```python
from build123d import *

# Parameters (mm, degrees)
SKETCH_1_R      = 1.5
EXTRUDE_1_DEPTH = 1.5
EXTRUDE_2_DEPTH = 5
SKETCH_3_R      = 6
EXTRUDE_3_DEPTH = 3
SKETCH_4_R      = 4
EXTRUDE_4_DEPTH = 5


with BuildPart() as part:
    # 草图1 → 凸台-拉伸1 (new body)
    with BuildSketch(Plane(origin=(0, 0, 0), x_dir=(1, 0, 0), z_dir=(0, 1, 0))):
        with BuildLine():
            Line((-11, 13.5), (11, 13.5))
            ThreePointArc((11, 13.5), (14.535533906, 12.035533906), (16, 8.5))
            Line((16, 8.5), (16, -5.5))
            ThreePointArc((16, -5.5), (13.656854249, -11.156854249), (8, -13.5))
            Line((8, -13.5), (-8, -13.5))
            ThreePointArc((-8, -13.5), (-13.656854249, -11.156854249), (-16, -5.5))
            Line((-16, -5.5), (-16, 8.5))
            ThreePointArc((-16, 8.5), (-14.535533906, 12.035533906), (-11, 13.5))
        make_face()
        with Locations(Location((-13.4, 8.5, 0), (0, 0, 270))):
            Circle(SKETCH_1_R, mode=Mode.SUBTRACT)
        with Locations(Location((13.5, 8.5, 0), (0, 0, 270))):
            Circle(SKETCH_1_R, mode=Mode.SUBTRACT)
        with Locations(Location((-13.4, -2.93, 0), (0, 0, 270))):
            Circle(SKETCH_1_R, mode=Mode.SUBTRACT)
        with Locations(Location((13.5, -2.93, 0), (0, 0, 270))):
            Circle(SKETCH_1_R, mode=Mode.SUBTRACT)
    extrude(amount=EXTRUDE_1_DEPTH)

    # 草图2 → 凸台-拉伸2 (add)
    with BuildSketch(Plane(origin=(0, 1.5, 0), x_dir=(1, 0, 0), z_dir=(0, 1, 0))):
        Polygon((-9, 11.5), (9, 11.5), (11, 9.5), (11, -5.5), (9, -7.5), (-9, -7.5), (-11, -5.5), (-11, 9.5), align=None)
    extrude(amount=EXTRUDE_2_DEPTH)

    # 草图3 → 凸台-拉伸3 (add)
    with BuildSketch(Plane(origin=(0, 6.5, 0), x_dir=(1, 0, 0), z_dir=(0, 1, 0))):
        with Locations(Location((0, 3.5, 0), (0, 0, 270))):
            Circle(SKETCH_3_R)
    extrude(amount=EXTRUDE_3_DEPTH)

    # 草图4 → 凸台-拉伸4 (add)
    with BuildSketch(Plane(origin=(0, 9.5, 0), x_dir=(1, 0, 0), z_dir=(0, 1, 0))):
        with Locations(Location((0, 3.5, 0), (0, 0, 270))):
            Circle(SKETCH_4_R)
    extrude(amount=EXTRUDE_4_DEPTH)


solid = part.part
```
Geometry: final body of the model. Coordinates: model frame, mm. A direction names the side the tool comes from. Round coordinates to 2 decimals unless told otherwise and drop trailing zeros. Order: outer loops, then holes, each group sorted by start corner. A loop starts at its lowest first (then second) coordinate and runs counter-clockwise, first axis right, second up. Notation, with made-up numbers: (-19, -39.75) - (30, -39.75) arc R14 ccw to (30, -23.75) - close; hole circle Ø10 at (22, -39). An arc over 180 degrees is marked (long way). Write item = value, one per line. Start each with the question number.
Q1. Cut plane C-C on x = 0. Return the cut outline in (y, z).
Q2. Ray query, line 1 (X direction, y = 0.85, z = -8.5); line 2 (Z direction, x = -12.5, y = 1); line 3 (Y direction, x = -10, z = -6). Return the intervals inside material, ascending. Write a range as from..to.
Q3. Cut plane A-A on y = 1. Return the cut outline in (x, z), and give its area (3 significant figures).
Q4. Pin query (flat end, axial travel): pin 1 (1.5 mm diameter, centred on y = 7, z = 4, fed in from -X); pin 2 (4 mm diameter, centred on y = 4, z = -2.5, fed in from +X); pin 3 (5.5 mm diameter, centred on x = -1.5, y = 4.5, fed in from -Z). Return the tip coordinate at first contact, or that it passes through.
Q5. Cut plane D-D on z = -3.5. Return the cut outline in (x, y), and give its area (3 significant figures).
Q6. Cut plane B-B on z = 2.93. Return the cut outline in (x, y).
Q7. Pull-direction query (X, two-part tool) for faces 6 (the cylindrical face through (-14.57, 0.74, -12)), 7 (the cylindrical face through (13.719, 0.74, 11.094)), 8 (the flat face through (0, 4, -11.5)), 9 (the cylindrical face through (13.57, 0.74, -10)); classes: +X half, -X half, draft (parallel to the pull), parting line (faces both ways), or undercut.
Q8. Access query for faces 1 (the flat face through (-11, 4, -2)), 2 (the flat face through (-10, 4, 6.5)), 3 (the flat face through (-10, 4, -10.5)), 4 (the flat face through (11, 4, -2)), 5 (the cylindrical face through (-2.4, 12, -6.7)). Directions: +Z, -Z, +X, -X, +Y, -Y. A direction counts if a zero-diameter tool reaches every point of the face in a straight line with its end or side. Return the directions, or none.
Outcome:
q1.outline = (0, -13.5) - (1.5, -13.5) - (1.5, -11.5) - (6.5, -11.5) - (6.5, -9.5) - (9.5, -9.5) - (9.5, -7.5) - (14.5, -7.5) - (14.5, 0.5) - (9.5, 0.5) - (9.5, 2.5) - (6.5, 2.5) - (6.5, 7.5) - (1.5, 7.5) - (1.5, 13.5) - (0, 13.5) - close
q2.line_1 = -16..-14.9, -11.9..12, 15..16
q2.line_2 = -13.27..-9.7, -7.3..1.73, 4.13..12.11
q2.line_3 = 0..6.5
q3.outline = (-16, -8.5) arc R5 ccw to (-11, -13.5) - (11, -13.5) arc R5 ccw to (16, -8.5) - (16, 5.5) arc R8 ccw to (8, 13.5) - (-8, 13.5) arc R8 ccw to (-16, 5.5) - close; hole circle Ø3 at (-13.4, -8.5); hole circle Ø3 at (-13.4, 2.93); hole circle Ø3 at (13.5, -8.5); hole circle Ø3 at (13.5, 2.93)
q3.area = 798 mm^2
q4.pin_1 = -11
q4.pin_2 = 11
q4.pin_3 = -11.5
q5.outline = (-16, 0) - (16, 0) - (16, 1.5) - (11, 1.5) - (11, 6.5) - (6, 6.5) - (6, 9.5) - (4, 9.5) - (4, 14.5) - (-4, 14.5) - (-4, 9.5) - (-6, 9.5) - (-6, 6.5) - (-11, 6.5) - (-11, 1.5) - (-16, 1.5) - close
q5.area = 234 mm^2
q6.outline = (-16, 0) - (-14.9, 0) - (-14.9, 1.5) - (-16, 1.5) - close; (-11.9, 0) - (12, 0) - (12, 1.5) - (11, 1.5) - (11, 6.5) - (-11, 6.5) - (-11, 1.5) - (-11.9, 1.5) - close; (15, 0) - (16, 0) - (16, 1.5) - (15, 1.5) - close
q7.face_6 = -X half
q7.face_7 = +X half
q7.face_8 = draft
q7.face_9 = undercut
q8.face_1 = +Z, -Z, -X, +Y
q8.face_2 = +Z, -X, +Y
q8.face_3 = -Z, -X, +Y
q8.face_4 = +Z, -Z, +X, +Y
q8.face_5 = +Y
